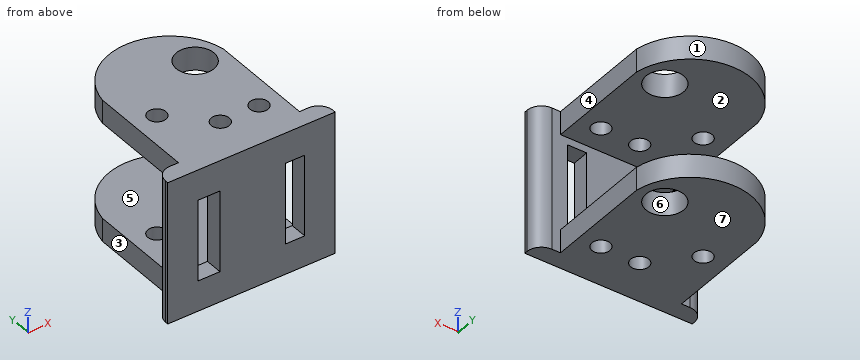
```python
from build123d import *

# Parameters (mm, degrees)
SKETCH2_R           = 1.5875
SKETCH2_R_2         = 3.302
BOSS_EXTRUDE1_DEPTH = 24.892
CUT_EXTRUDE2_DEPTH  = 21.844
SKETCH4_W           = 3.326504507
SKETCH4_H           = 14.224
SKETCH4_W_2         = 3.81
CUT_EXTRUDE3_DEPTH  = 21.844
FILLET1_R           = 2.54


with BuildPart() as part:
    # Sketch2 → Boss-Extrude1 (new body)
    with BuildSketch(Plane.XY):
        with BuildLine():
            Line((8.660504507, -21.669967929), (-20.659495493, -21.669967929))
            Line((-20.659495493, -21.669967929), (-20.659495493, -18.621967929))
            Line((-20.659495493, -18.621967929), (-16.595495493, -18.621967929))
            Line((-16.595495493, -18.621967929), (-16.595495493, -0.055984768))
            ThreePointArc((-16.595495493, -0.055984768), (-5.999495493, 8.944015232), (4.596504507, -0.055984768))
            Line((4.596504507, -0.055984768), (4.596504507, -18.621967929))
            Line((4.596504507, -18.621967929), (8.660504507, -18.621967929))
            Line((8.660504507, -18.621967929), (8.660504507, -21.669967929))
        make_face()
        with Locations((-12.446, -7.546743134)):
            Circle(SKETCH2_R, mode=Mode.SUBTRACT)
        with Locations((-0.339495493, 0)):
            Circle(SKETCH2_R_2, mode=Mode.SUBTRACT)
        with Locations((-5.999495493, -14.049967929)):
            Circle(SKETCH2_R, mode=Mode.SUBTRACT)
        with Locations((0.786504507, -14.049967929)):
            Circle(SKETCH2_R, mode=Mode.SUBTRACT)
    extrude(amount=BOSS_EXTRUDE1_DEPTH)

    # Sketch3 → Cut-Extrude2 (cut)
    with BuildSketch(Plane.ZY.offset(16.595495493)):
        Polygon((20.828, -18.621967929), (20.828, 11.195500081), (4.064, 11.195500081), (4.064, -0.055984768), (4.064, -18.621967929), align=None)
    extrude(amount=-CUT_EXTRUDE2_DEPTH, mode=Mode.SUBTRACT)

    # Sketch4 → Cut-Extrude3 (cut)
    with BuildSketch(Plane(origin=(0, -18.621967929, 0), x_dir=(1, 0, 0), z_dir=(0, 1, 0))):
        with Locations((1.663252254, -12.446)):
            Rectangle(SKETCH4_W, SKETCH4_H)
        with Locations((-13.420495493, -12.446)):
            Rectangle(SKETCH4_W_2, SKETCH4_H)
    extrude(amount=-CUT_EXTRUDE3_DEPTH, mode=Mode.SUBTRACT)

    # Fillet1
    fillet1_edges = [part.edges().sort_by_distance(p)[0] for p in [
        (-20.659495493, -18.621967929, 12.446),
        (8.660504507, -18.621967929, 12.446),
    ]]
    fillet(fillet1_edges, radius=FILLET1_R)


solid = part.part
```
Here's how the part is built. I have some questions about the finished solid (model axes, mm). Face numbers are marked on the shaded views. A direction names the side the tool comes from. Coordinates: 2 decimals unless noted, no trailing zeros. Order: outer loops, then holes, each group sorted by start corner. A loop starts at its lowest first (then second) coordinate and runs counter-clockwise, first axis right, second up. Notation, with made-up numbers: M 26.25,-25.75 L 51.25,-25.75 A32 ccw 51.25,8.25 Z; hole C 12,-5.5 d11. An arc over 180 degrees is marked long. Answer as a JSON object with one key per item and string values. Group by question number.
(1) Suppose I cut it at C-C, the plane x = 0.5. Please give me the cut outline in (y, z).
(2) Suppose I cut it at A-A, the plane y = -10. Please give me the cut outline in (x, z), then the cut area to 3 significant figures.
(3) Suppose I cut it at D-D, the plane x = -7. Please give me the cut outline in (y, z).
(4) If we mould it in two halves opening along Z, with no side actions, what happens to the marked faces 5, 6 and 7? For each: released by +Z, released by -Z, zero draft, split by the parting line, or undercut.
(5) I need wall thicknesses on probe 1 along Z at (x, y) = (-5.5, 1); probe 2 along Y at (x, z) = (4, 7.75); probe 3 along X at (y, z) = (-1.5, 1.5). Which ranges of each line are inside material? Lowest first, please.
(6) Which directions (+Z, -Z, +X, -X, +Y, -Y) give clear straight access to the entire face, cutting with the end or side of a thin tool? Please do the marked faces 1, 2, 3 and 4.
(7) Suppose I cut it at B-B, the plane z = 6.25. Please give me the cut outline in (x, y).
(8) For pin 1 (2 mm diameter, centred on y = -5, z = 23, fed in from -X); pin 2 (8 mm diameter, centred on y = -3, z = 5, fed in from +X); pin 3 (7.5 mm diameter, centred on x = -10, z = 16, fed in from +Y), each with a flat end and sliding along its axis, tell me the tip position at first contact or that it passes through.
Values found:
{
 "1": {"outline": "M -21.67,0 L -15.61,0 L -15.61,4.06 L -18.62,4.06 L -18.62,5.33 L -21.67,5.33 Z; M -21.67,19.56 L -18.62,19.56 L -18.62,20.83 L -15.61,20.83 L -15.61,24.89 L -21.67,24.89 Z; M -12.49,0 L -3.19,0 L -3.19,4.06 L -12.49,4.06 Z; M -12.49,20.83 L -3.19,20.83 L -3.19,24.89 L -12.49,24.89 Z; M 3.19,0 L 6.75,0 L 6.75,4.06 L 3.19,4.06 Z; M 3.19,20.83 L 6.75,20.83 L 6.75,24.89 L 3.19,24.89 Z"},
 "2": {"outline": "M -16.6,0 L 4.6,0 L 4.6,4.06 L -16.6,4.06 Z; M -16.6,20.83 L 4.6,20.83 L 4.6,24.89 L -16.6,24.89 Z", "area": "172 mm^2"},
 "3": {"outline": "M -21.67,0 L -15.28,0 L -15.28,4.06 L -18.62,4.06 L -18.62,20.83 L -15.28,20.83 L -15.28,24.89 L -21.67,24.89 Z; M -12.82,0 L 8.9,0 L 8.9,4.06 L -12.82,4.06 Z; M -12.82,20.83 L 8.9,20.83 L 8.9,24.89 L -12.82,24.89 Z"},
 "4": {"face 5": "undercut", "face 6": "zero draft", "face 7": "released by -Z"},
 "5": {"probe 1": "z = 0 to 4.06, 20.83 to 24.89", "probe 2": "y = -21.67 to -18.62", "probe 3": "x = -16.6 to -3.28, 2.6 to 4.6"},
 "6": {"face 1": "+Z, -Z, +Y", "face 2": "+X, -X, +Y", "face 3": "+Z, -Z, -X, +Y", "face 4": "+Z, -Z, +X, +Y"},
 "7": {"outline": "M -20.66,-21.67 L -15.33,-21.67 L -15.33,-18.62 L -18.12,-18.62 A2.54 ccw -20.66,-21.16 Z; M -11.52,-21.67 L 0,-21.67 L 0,-18.62 L -11.52,-18.62 Z; M 3.33,-21.67 L 8.66,-21.67 L 8.66,-21.16 A2.54 ccw 6.12,-18.62 L 3.33,-18.62 Z"},
 "8": {"pin 1": "stops at x = -16.6", "pin 2": "stops at x = 4.6", "pin 3": "stops at y = -18.62"}
}
